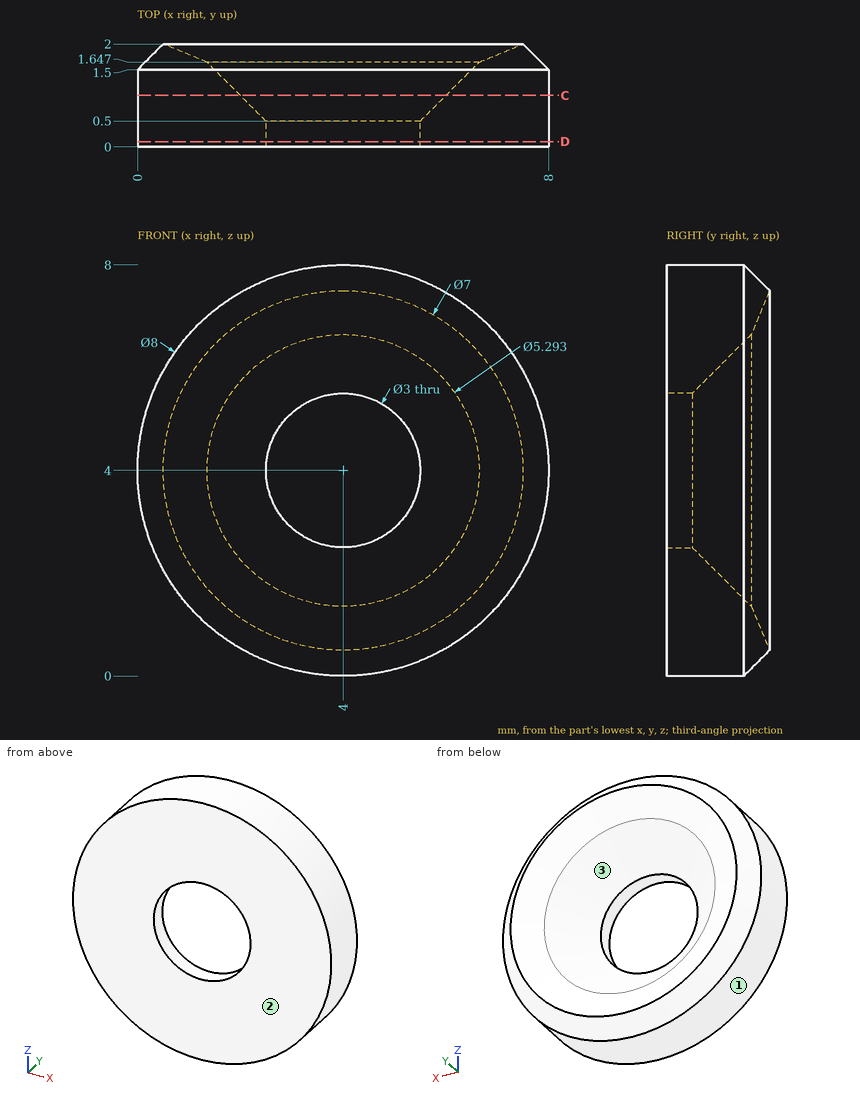
Could you check a few things on this drawing? It's one solid part, dimensions in mm from its lowest x, y, z. Round coordinates to 2 decimals unless told otherwise and drop trailing zeros. Write each loop counter-clockwise with the first axis right and the second up, starting at its lowest first coordinate (ties: lowest second). Pieces come first, ordered by that corner, then holes.
Q1. If we mould it in two halves opening along Z, with no side actions, what happens to the marked faces 1, 2 and 3? For each: +Z half, -Z half, draft (parallel to the pull), parting line (faces both ways), or undercut.
Q2. If we section it at C-C on y = 1: Write out the boundary of the cut face in (x, z), plus the area to 3 significant figures.
Q3. Please list where these lines run through material, in increasing order: probe 1 along X at (y, z) = (0.35, 4); probe 2 along X at (y, z) = (1.05, 2.75) (1 decimal); probe 3 along Z at (x, y) = (5.25, 1.15).
Q4. Will this pin go through, and if not, where does the flat tip stop? P1, Ø1, axis at y = 1, z = 1.5, coming from the +X side (1 decimal).
Q5. If we section it at D-D on y = 0.1: Write out the boundary of the cut face in (x, z), plus the area to 3 significant figures.
Answer below:
1. face 1: parting line
1. face 2: draft
1. face 3: undercut
2. outline: circle Ø8 at (4, 4); hole circle Ø4 at (4, 4)
2. area: 37.7 mm2
3. probe 1: x = 0 to 2.5, 5.5 to 8
3. probe 2: x = 0.2 to 2.4, 5.6 to 7.8
3. probe 3: z = 0.2 to 2.25, 5.75 to 7.8
4. P1: stops at x = 7.5
5. outline: circle Ø8 at (4, 4); hole circle Ø3 at (4, 4)
5. area: 43.2 mm2
